Can you work these out from the model? Positions are in its coordinate system, mm. A direction names the side the tool comes from. Coordinates: 2 decimals unless noted, no trailing zeros. Order: outer loops, then holes, each group sorted by start corner. A loop starts at its lowest first (then second) coordinate and runs counter-clockwise, first axis right, second up. Notation, with made-up numbers: (34.5, 73.25) -> (44.5, 73.25) arc R29 ccw to (44.5, 108.25) -> close; hole circle Ø11 at (65.25, 87.25). An arc over 180 degrees is marked (long way). Answer in a Markdown table with one row per item. Add a question column.
1. On a 3-axis mill with a long thin cutter (end or side, diameter ignored), from which of +Z, -Z, +X, -X, +Y, -Y can I reach the whole of each face in a straight line? I mean faces 1 (the face through (-19.05, -6, 67)), 2 (the face through (14, -6, 63.5)), 3 (the face through (-31.75, -6, 3)), 4 (the face through (14, -6, 69.85)), 5 (the face through (-24.9, -6.26, 35.33)). Say none if no direction works.
2. We'd pull the mould along X, two halves only. Please class faces 6 (the face through (2.56, -6.26, 62.66)), 7 (the face through (50.8, -6, 3)), 8 (the face through (-46, -6, 6.35)): pulls with the +X half, pulls with the -X half, needs draft (parallel to the pull), parting line crosses it, or undercut.
3. If I drill on line 1 along Z through (x, y) = (0, -2.5); line 2 along X through (y, z) = (-4.5, 67); line 3 along X through (y, z) = (-9.5, 70), over which ranges is the centre line in solid material (lowest first)? Write a range as [from, to].
4. Will these pins go through, and if not, where does the flat tip stop? pin 1 (5 mm diameter, centred on x = -13, y = -7.5, fed in from +Z); pin 2 (3 mm diameter, centred on x = -46.5, y = -4.5, fed in from +Z); pin 3 (7 mm diameter, centred on y = -6.5, z = 68, fed in from +X).
5. Imagine slicing it at C-C on z = 55. Write out the boundary of the cut face in (x, y), plus the area to 3 significant figures.
6. Imagine slicing it at A-A on x = 0. Write out the boundary of the cut face in (y, z).
7. Imagine slicing it at D-D on x = -21.5. Write out the boundary of the cut face in (y, z) (3 decimals).
from build123d import *

# Parameters (mm, degrees)
F1_DEPTH = 12.7
F2_DEPTH = 12.7


with BuildPart() as f1:
    # F0 (on Front) → F1 (new body)
    with BuildSketch(Plane.XZ):
        with BuildLine():
            Line((-50.8, 6.35), (-50.8, 0))
            Line((-50.8, 0), (-31.75, 0))
            Line((-31.75, 0), (-31.75, 6.35))
            Line((-31.75, 6.35), (-19.920041, 28.826923))
            ThreePointArc((-19.920041, 28.826923), (0, 40.194522), (19.920041, 28.826923))
            Line((19.920041, 28.826923), (31.75, 6.35))
            Line((31.75, 6.35), (31.75, 0))
            Line((31.75, 0), (50.8, 0))
            Line((50.8, 0), (50.8, 6.35))
            Line((50.8, 6.35), (41.275, 6.35))
            Line((41.275, 6.35), (8.980256, 63.5))
            Line((8.980256, 63.5), (19.05, 63.5))
            Line((19.05, 63.5), (19.05, 66.675))
            Line((19.05, 66.675), (9.525, 66.675))
            Line((9.525, 66.675), (4.7625, 66.675))
            ThreePointArc((4.7625, 66.675), (0, 61.9125), (-4.7625, 66.675))
            Line((-4.7625, 66.675), (-9.525, 66.675))
            Line((-9.525, 66.675), (-19.05, 66.675))
            Line((-19.05, 66.675), (-19.05, 63.5))
            Line((-19.05, 63.5), (-8.980256, 63.5))
            Line((-8.980256, 63.5), (-41.275, 6.35))
            Line((-41.275, 6.35), (-50.8, 6.35))
        make_face()
    extrude(amount=F1_DEPTH)

    # F0 (on Front) → F2 (join)
    with BuildSketch(Plane.XZ):
        with BuildLine():
            Line((-19.05, 69.85), (-19.05, 66.675))
            Line((-19.05, 66.675), (-9.525, 66.675))
            Line((-9.525, 66.675), (-4.7625, 66.675))
            ThreePointArc((-4.7625, 66.675), (0, 71.4375), (4.7625, 66.675))
            Line((4.7625, 66.675), (9.525, 66.675))
            Line((9.525, 66.675), (19.05, 66.675))
            Line((19.05, 66.675), (19.05, 69.85))
            Line((19.05, 69.85), (8.980256, 69.85))
            ThreePointArc((8.980256, 69.85), (0, 76.2), (-8.980256, 69.85))
            Line((-8.980256, 69.85), (-19.05, 69.85))
        make_face()
    extrude(amount=F2_DEPTH)


solid = f1.part
Answers follow:
| question | item | result |
|---|---|---|
| 1 | face 1 | +Z, -X, +Y, -Y |
| 1 | face 2 | +X, +Y, -Y |
| 1 | face 3 | -Z, +Y, -Y |
| 1 | face 4 | +Z, +X, +Y, -Y |
| 1 | face 5 | -X, +Y, -Y |
| 2 | face 6 | undercut |
| 2 | face 7 | pulls with the +X half |
| 2 | face 8 | needs draft |
| 3 | line 1 | z = [40.19, 61.91], [71.44, 76.2] |
| 3 | line 2 | x = [-19.05, -4.75], [4.75, 19.05] |
| 3 | line 3 | x = [-8.93, -3.41], [3.41, 8.93] |
| 4 | pin 1 | stops at z = 69.85 |
| 4 | pin 2 | stops at z = 6.35 |
| 4 | pin 3 | stops at x = 19.05 |
| 5 | outline | (-13.78, -12.7) -> (13.78, -12.7) -> (13.78, 0) -> (-13.78, 0) -> close |
| 5 | area | 350 mm² |
| 6 | outline | (-12.7, 40.19) -> (0, 40.19) -> (0, 61.91) -> (-12.7, 61.91) -> close; (-12.7, 71.44) -> (0, 71.44) -> (0, 76.2) -> (-12.7, 76.2) -> close |
| 7 | outline | (-12.7, 25.825) -> (0, 25.825) -> (0, 41.345) -> (-12.7, 41.345) -> close |
